For this review, take the finished solid that the model builds, in its own axes (mm). A direction names the side the tool comes from. Give positions to 0.01 mm unless a question says otherwise; leave off trailing zeros. Write each loop counter-clockwise with the first axis right and the second up, starting at its lowest first coordinate (ties: lowest second). Pieces come first, ordered by that corner, then holes.
Q1. Machinability: for faces 4 (the flat face through (2, 90, 2)), 5 (the flat face through (130, 140, 3)), 6 (the flat face through (213, 72, 3)), 7 (the flat face through (232, 145, 2)), which of the approach directions +Z, -Z, +X, -X, +Y, -Y give a long, thin tool a straight path to every point of the face, cutting with its end or side? Answer none if there is none.
Q2. We need section A-A (x = 202.5). Write out the cut boundary in (y, z).
Q3. Mouldability with a two-part tool opening along Y and no side actions: class faces 1 (the flat face through (215, 91.8, 3)), 2 (the flat face through (5, 18, 2)), 3 (the flat face through (3, 120, 2)) as released by +Y, released by -Y, zero draft, split by the parting line, or undercut.
Q4. We need section D-D (y = 85). Write out the cut boundary in (x, z).
Q5. We need section C-C (x = 127.5). Write out the cut boundary in (y, z), then the cut area to 3 significant figures.
Q6. For line 1 (Y direction, x = 215, z = 4); line 2 (X direction, y = 78.5, z = 1); line 3 (Y direction, x = 97.5, z = 1.95), list the stretches that pass through material, from the lowest coordinate up.
Q7. Insertion check: P1, Ø1.5, axis at y = 71.5, z = 3.5, coming from the -X side; P2, Ø2.5, axis at y = 147.5, z = 1.5, coming from the -X side; P3, Ø1.5, axis at x = 131.5, z = 3.5, coming from the -Y side; P4, Ø2, axis at x = 79.5, z = 1, coming from the -Y side. Each pin has a flat end and moves straight along its axis. Give the tip position at first contact, or say it passes through.
Q8. We need section B-B (y = 41). Write out the cut boundary in (x, z).
```python
from build123d import *

# Parameters (mm, degrees)
SALIENTE_EXTRUIR1_DEPTH = 5
CROQUIS2_W              = 52
CROQUIS2_H              = 5
CORTAR_EXTRUIR1_DEPTH   = 10
CROQUIS3_W              = 5
CROQUIS3_H              = 38.6
CROQUIS3_W_2            = 156
CROQUIS3_H_2            = 95.8
CORTAR_EXTRUIR2_DEPTH   = 10


with BuildPart() as part:
    # Croquis1 → Saliente-Extruir1 (new body)
    with BuildSketch(Plane.XY):
        Polygon((52, 0), (104, 0), (104, 5), (156, 5), (156, 0), (208, 0), (208, 5), (255, 5), (255, 30), (260, 30), (260, 60), (255, 60), (255, 90), (260, 90), (260, 120), (255, 120), (255, 145), (208, 145), (208, 150), (156, 150), (156, 145), (104, 145), (104, 150), (52, 150), (52, 145), (5, 145), (5, 120), (0, 120), (0, 90), (5, 90), (5, 60), (0, 60), (0, 30), (5, 30), (5, 5), (52, 5), align=None)
    extrude(amount=SALIENTE_EXTRUIR1_DEPTH)

    # Croquis2 → Cortar-Extruir1 (cut)
    with BuildSketch(Plane.XY.offset(5)):
        with Locations((130, 142.5)):
            Rectangle(CROQUIS2_W, CROQUIS2_H)
    extrude(amount=-CORTAR_EXTRUIR1_DEPTH, mode=Mode.SUBTRACT)

    # Croquis3 → Cortar-Extruir2 (cut)
    with BuildSketch(Plane.XY.offset(5)):
        with Locations((44.5, 72.5)):
            Rectangle(CROQUIS3_W, CROQUIS3_H)
        with Locations((130, 72.5)):
            Rectangle(CROQUIS3_W_2, CROQUIS3_H_2)
        Polygon((47, 19.6), (100.666666667, 19.6), (100.666666667, 14.6), (42, 14.6), (42, 19.6), align=None)
        with Locations((215.5, 72.5)):
            Rectangle(CROQUIS3_W, CROQUIS3_H)
        Polygon((47, 125.4), (100.666666667, 125.4), (100.666666667, 130.4), (42, 130.4), (42, 125.4), align=None)
        Polygon((218, 130.4), (218, 125.4), (213, 125.4), (159.333333333, 125.4), (159.333333333, 130.4), align=None)
        Polygon((159.333333333, 14.6), (159.333333333, 19.6), (213, 19.6), (218, 19.6), (218, 14.6), align=None)
    extrude(amount=-CORTAR_EXTRUIR2_DEPTH, mode=Mode.SUBTRACT)


solid = part.part
```
Computed:
1. face 4: +Z, -Z, -X
1. face 5: +Z, -Z, +Y
1. face 6: +Z, -Z
1. face 7: +Z, -Z, +X, +Y
2. outline: (0, 0) - (14.6, 0) - (14.6, 5) - (0, 5) - close; (19.6, 0) - (24.6, 0) - (24.6, 5) - (19.6, 5) - close; (120.4, 0) - (125.4, 0) - (125.4, 5) - (120.4, 5) - close; (130.4, 0) - (150, 0) - (150, 5) - (130.4, 5) - close
3. face 1: undercut
3. face 2: zero draft
3. face 3: released by +Y
4. outline: (5, 0) - (42, 0) - (42, 5) - (5, 5) - close; (47, 0) - (52, 0) - (52, 5) - (47, 5) - close; (208, 0) - (213, 0) - (213, 5) - (208, 5) - close; (218, 0) - (255, 0) - (255, 5) - (218, 5) - close
5. outline: (5, 0) - (24.6, 0) - (24.6, 5) - (5, 5) - close; (120.4, 0) - (140, 0) - (140, 5) - (120.4, 5) - close
5. area: 196 mm2
6. line 1: y = 5 to 14.6, 19.6 to 53.2, 91.8 to 125.4, 130.4 to 145
6. line 2: x = 5 to 42, 47 to 52, 208 to 213, 218 to 255
6. line 3: y = 0 to 14.6, 19.6 to 24.6, 120.4 to 125.4, 130.4 to 150
7. P1: stops at x = 5
7. P2: stops at x = 52
7. P3: stops at y = 5
7. P4: stops at y = 0
8. outline: (0, 0) - (52, 0) - (52, 5) - (0, 5) - close; (208, 0) - (260, 0) - (260, 5) - (208, 5) - close
